Geometry check sheet. Reference: drawing and pictorial views, mm from the part's lowest x, y, z. A direction names the side the tool comes from. Round coordinates to 2 decimals unless told otherwise and drop trailing zeros. Loops run counter-clockwise (first coordinate to the right, second up) from the corner with the lowest first, then second, coordinate; pieces in that order, holes last. Notation, with made-up numbers: (57, -13.5) -> (65, -13.5) arc R26 ccw to (65, 15.5) -> close; hole circle Ø2 at (-7.75, -29). An arc over 180 degrees is marked (long way). Use one line per item in the form item = value. Start each with the question number.
(1) Go/stop test with flat-tipped pins: pin 1 (1.5 mm diameter, centred on y = 9.5, z = 8, fed in from +X); pin 2 (4 mm diameter, centred on x = 9, z = 14, fed in from -Y); pin 3 (1.5 mm diameter, centred on x = 10.5, y = 41, fed in from -Z); pin 4 (7.5 mm diameter, centred on x = 7.5, z = 18, fed in from -Y). Record where each tip stops, or that it passes through.
(2) Sectioned sample at B-B (x = 3.25). Record the cut outline in (y, z), and give its area (3 significant figures).
(3) Set-up check for the marked faces 1, 2, 3 and 4: record each of +Z, -Z, +X, -X, +Y, -Y from which the full face is reachable in a straight line by a thin tool's end or side.
(4) Sectioned sample at D-D (y = 35). Record the cut outline in (x, z).
(5) Draft check along Y on the marked faces 5, 6 and 7. Enter one of: released by +Y, released by -Y, zero draft, split by the parting line, or undercut.
(6) Material ranges on probe 1 along Y at (x, z) = (10, 25); probe 2 along X at (y, z) = (18, 17); probe 3 along Z at (x, y) = (21.75, 49), recorded low to high. Write a range as [from, to].
(7) Sectioned sample at A-A (y = 50). Record the cut outline in (x, z), and give its area (3 significant figures).
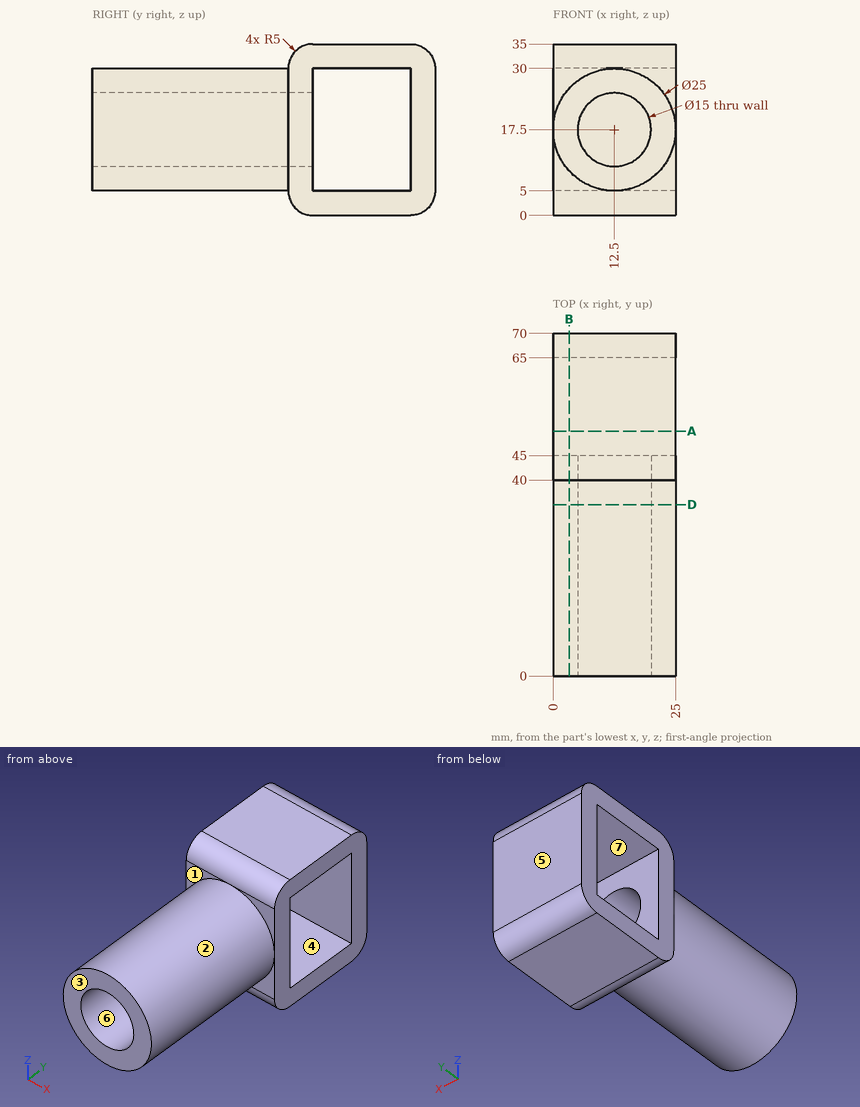
Checks:
q1.pin_1 = 21.43
q1.pin_2 = 65
q1.pin_3 = 1.2
q1.pin_4 = 0
q2.outline = (0, 9.09) -> (40, 9.09) -> (40, 5) arc R5 ccw to (45, 0) -> (65, 0) arc R5 ccw to (70, 5) -> (70, 30) arc R5 ccw to (65, 35) -> (45, 35) arc R5 ccw to (40, 30) -> (40, 25.91) -> (0, 25.91) -> close; hole (45, 5) -> (65, 5) -> (65, 30) -> (45, 30) -> close
q2.area = 1,200 mm2
q3.face_1 = +Z, -Y
q3.face_2 = -Y
q3.face_3 = +Z, -Z, +X, -X, -Y
q3.face_4 = +X, -X
q4.outline = circle Ø25 at (12.5, 17.5); hole circle Ø15 at (12.5, 17.5)
q5.face_5 = released by +Y
q5.face_6 = zero draft
q5.face_7 = undercut
q6.probe_1 = [0, 45], [65, 70]
q6.probe_2 = [0.01, 5.02], [19.98, 24.99]
q6.probe_3 = [0, 5], [30, 35]
q7.outline = (0, 0) -> (25, 0) -> (25, 5) -> (0, 5) -> close; (0, 30) -> (25, 30) -> (25, 35) -> (0, 35) -> close
q7.area = 250 mm2
